Geometry: final body of the model. Coordinates: model frame, mm. Face numbers are marked on the shaded views. A direction names the side the tool comes from. Give positions to 0.01 mm unless a question says otherwise; leave off trailing zeros. Order: outer loops, then holes, each group sorted by start corner. A loop starts at its lowest first (then second) coordinate and runs counter-clockwise, first axis right, second up. Notation, with made-up numbers: (89, -21.5) -> (114, -21.5) arc R22 cw to (114, 12.5) -> close; hole circle Ø7 at (33, -2.5). An arc over 180 degrees is marked (long way). Answer in a Markdown table with one row per item. Add a question column.
Q1. Line query: line 1 along X through (y, z) = (-2.95, 52); line 2 along Y through (x, z) = (17, 6); line 3 along Y through (x, z) = (22, 5). Output: solid intervals per line, ascending. Write a range as from..to.
Q2. Cut plane D-D on y = 23. Return the cut outline in (x, z).
Q3. Cut plane C-C on z = 55. Return the cut outline in (x, y).
Q4. Cut plane A-A on x = 10. Return the cut outline in (y, z), and give its area (3 significant figures).
Q5. Cut plane B-B on y = 10.1. Return the cut outline in (x, z).
Q6. Pull-direction query (Y, two-part tool) for the marked faces 3, 4 and 5; classes: +Y half, -Y half, draft (parallel to the pull), parting line (faces both ways), or undercut.
Q7. Set-up query: the marked faces 1 and 2. Return all of +Z, -Z, +X, -X, +Y, -Y with unobstructed straight access to the full face (end or side cutting, diameter ignored); none if empty.
Q8. Contact query for flat-ended pins moving along their axis: P1, Ø5, axis at y = 10.1, z = 5, coming from the -X side (1 decimal); P2, Ø4.5, axis at y = 13, z = 8.5, coming from the -X side; P3, Ø10, axis at y = 8, z = 38.5, coming from the -X side; P4, Ø1, axis at x = 25.5, y = 20.5, coming from the -Z side. Output: stop coordinate, or through.
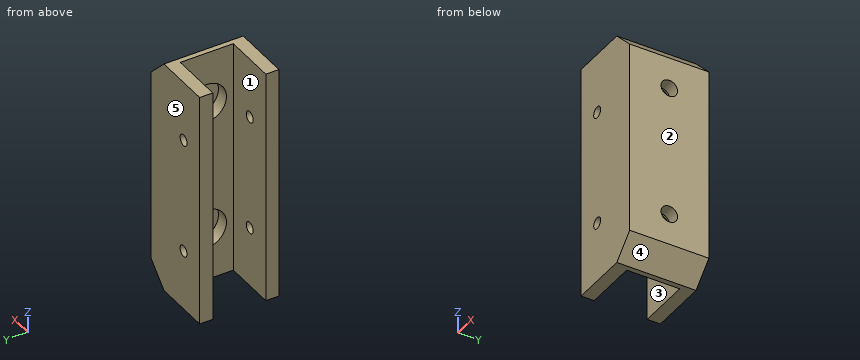
from build123d import *

# Parameters (mm, degrees)
EXTRUDE_1_DEPTH     = 60
SKETCH_4_R          = 2.15
CUT_EXTRUDE_1_DEPTH = 40
SKETCH_5_R          = 3.15
CUT_EXTRUDE_2_DEPTH = 40
EXTRUDE_6_DEPTH     = 15
EXTRUDE_7_DEPTH     = 15
EXTRUDE_START       = 5
SKETCH_12_W         = 90
SKETCH_12_H         = 30.2
SKETCH_12_R         = 3.15
EXTRUDE_8_DEPTH     = 5
CHAMFER_6_SIZE      = 8
SKETCH_13_R         = 7.5
CUT_EXTRUDE_5_DEPTH = 5


with BuildPart() as part:
    # 草图1 → 凸台-拉伸1 (new body)
    with BuildSketch(Plane.XY):
        Polygon((0, 0), (0, -5), (25.2, -5), (25.2, 25.2), (0, 25.2), (0, 20.2), (20.2, 20.2), (20.2, 0), align=None)
    extrude(amount=EXTRUDE_1_DEPTH)

    # 草图4 → 切除-拉伸1 (cut)
    with BuildSketch(Plane(origin=(0, 25.2, 0), x_dir=(1, 0, 0), z_dir=(0, 1, 0))):
        with Locations(Location((10, -8, 0), (0, 0, 270))):
            Circle(SKETCH_4_R)
        with Locations(Location((10, -52, 0), (0, 0, 270))):
            Circle(SKETCH_4_R)
    extrude(amount=-CUT_EXTRUDE_1_DEPTH, mode=Mode.SUBTRACT)

    # 草图5 → 切除-拉伸2 (cut)
    with BuildSketch(Plane(origin=(25.2, 0, 0), x_dir=(0, 0, -1), z_dir=(1, 0, 0))):
        with Locations(Location((-55, 10.1, 0), (0, 0, 90))):
            Circle(SKETCH_5_R)
        with Locations(Location((-5, 10.1, 0), (0, 0, 90))):
            Circle(SKETCH_5_R)
    extrude(amount=-CUT_EXTRUDE_2_DEPTH, mode=Mode.SUBTRACT)

    # 草图10 → 凸台-拉伸6 (add)
    with BuildSketch(Plane(origin=(0, 0, 0), x_dir=(-1, 0, 0), z_dir=(0, 0, -1))):
        Polygon((-20.2, 20.2), (0, 20.2), (0, 25.2), (-25.2, 25.2), (-25.2, -5), (0, -5), (0, 0), (-20.2, 0), align=None)
    extrude(amount=EXTRUDE_6_DEPTH)

    # 草图11 → 凸台-拉伸7 (add)
    with BuildSketch(Plane.XY.offset(60)):
        Polygon((20.2, 0), (0, 0), (0, -5), (25.2, -5), (25.2, 25.2), (0, 25.2), (0, 20.2), (20.2, 20.2), align=None)
    extrude(amount=EXTRUDE_7_DEPTH)

    # 草图12 → 凸台-拉伸8 (add)
    with BuildSketch(Plane(origin=(25.2, 0, 0), x_dir=(0, 0, -1), z_dir=(1, 0, 0)).offset(EXTRUDE_START)):
        with Locations((-30, 10.1)):
            Rectangle(SKETCH_12_W, SKETCH_12_H)
        with Locations(Location((-55, 10.1, 0), (0, 0, 90))):
            Circle(SKETCH_12_R, mode=Mode.SUBTRACT)
        with Locations(Location((-5, 10.1, 0), (0, 0, 90))):
            Circle(SKETCH_12_R, mode=Mode.SUBTRACT)
    extrude(amount=-EXTRUDE_8_DEPTH)

    # 倒角6
    chamfer_6_edges = [part.edges().sort_by_distance(p)[0] for p in [
        (30.2, 10.1, -15),
        (30.2, 10.1, 75),
    ]]
    chamfer(chamfer_6_edges, length=CHAMFER_6_SIZE)

    # 草图13 → 切除-拉伸5 (cut)
    with BuildSketch(Plane.ZY.offset(-20.2)):
        with Locations((5, 10.1)):
            Circle(SKETCH_13_R)
        with Locations((55, 10.1)):
            Circle(SKETCH_13_R)
    extrude(amount=-CUT_EXTRUDE_5_DEPTH, mode=Mode.SUBTRACT)


solid = part.part
Completed:
| question | item | result |
|---|---|---|
| 1 | line 1 | x = 0..7.85, 12.15..30.2 |
| 1 | line 2 | y = -5..0, 20.2..25.2 |
| 1 | line 3 | y = -5..2.6, 17.6..25.2 |
| 2 | outline | (0, -15) -> (22.2, -15) -> (30.2, -7) -> (30.2, 67) -> (22.2, 75) -> (0, 75) -> close; hole circle Ø4.3 at (10, 8); hole circle Ø4.3 at (10, 52) |
| 3 | outline | (0, -5) -> (30.2, -5) -> (30.2, 6.95) -> (25.2, 6.95) -> (25.2, 2.6) -> (20.2, 2.6) -> (20.2, 0) -> (0, 0) -> close; (0, 20.2) -> (20.2, 20.2) -> (20.2, 17.6) -> (25.2, 17.6) -> (25.2, 13.25) -> (30.2, 13.25) -> (30.2, 25.2) -> (0, 25.2) -> close |
| 4 | outline | (-5, -15) -> (0, -15) -> (0, 5.85) -> (-5, 5.85) -> close; (-5, 10.15) -> (0, 10.15) -> (0, 49.85) -> (-5, 49.85) -> close; (-5, 54.15) -> (0, 54.15) -> (0, 75) -> (-5, 75) -> close; (20.2, -15) -> (25.2, -15) -> (25.2, 5.85) -> (20.2, 5.85) -> close; (20.2, 10.15) -> (25.2, 10.15) -> (25.2, 49.85) -> (20.2, 49.85) -> close; (20.2, 54.15) -> (25.2, 54.15) -> (25.2, 75) -> (20.2, 75) -> close |
| 4 | area | 814 mm² |
| 5 | outline | (20.2, -15) -> (22.2, -15) -> (30.2, -7) -> (30.2, 1.85) -> (25.2, 1.85) -> (25.2, -2.5) -> (20.2, -2.5) -> close; (20.2, 12.5) -> (25.2, 12.5) -> (25.2, 8.15) -> (30.2, 8.15) -> (30.2, 51.85) -> (25.2, 51.85) -> (25.2, 47.5) -> (20.2, 47.5) -> close; (20.2, 62.5) -> (25.2, 62.5) -> (25.2, 58.15) -> (30.2, 58.15) -> (30.2, 67) -> (22.2, 75) -> (20.2, 75) -> close |
| 6 | face 3 | undercut |
| 6 | face 4 | draft |
| 6 | face 5 | +Y half |
| 7 | face 1 | +Z, -Z, -X |
| 7 | face 2 | +Z, -Z, +X, +Y, -Y |
| 8 | P1 | passes through |
| 8 | P2 | stops at x = 25.2 |
| 8 | P3 | stops at x = 20.2 |
| 8 | P4 | stops at z = -12.2 |
